```python
from build123d import *

# Parameters (mm, degrees)
CYLINDER_R      = 20
CYLINDER_DEPTH  = 3.3
SKETCH_R        = 1.5
POCKET_DEPTH    = 3.301
POCKET001_DEPTH = 5


with BuildPart() as part:
    # Cylinder → Cylinder (new body)
    with BuildSketch(Plane.XY):
        Circle(CYLINDER_R)
    extrude(amount=CYLINDER_DEPTH)

    # Sketch (on Face2 of Cylinder) → Pocket (cut, through all)
    with BuildSketch(Plane.XY.offset(3.3)):
        with Locations((0, 15.1)):
            Circle(SKETCH_R)
    extrude(amount=-POCKET_DEPTH, mode=Mode.SUBTRACT)

    # CopySketch001 → Pocket001 (cut)
    with BuildSketch(Plane.XY.offset(3.3)):
        Polygon((8.911401, 5.145), (0, 10.29), (-8.911401, 5.145), (-8.911401, -5.145), (0, -10.29), (8.911401, -5.145), align=None)
    extrude(amount=-POCKET001_DEPTH, mode=Mode.SUBTRACT)


solid = part.part
```
The model under review builds one solid part; all positions refer to its coordinate system, in mm. A direction names the side the tool comes from. Coordinates: 2 decimals unless noted, no trailing zeros. Write each loop counter-clockwise with the first axis right and the second up, starting at its lowest first coordinate (ties: lowest second). Pieces come first, ordered by that corner, then holes. Notation, with made-up numbers: (70.5, 83) - (96.5, 83) arc R21 cw to (96.5, 110) - close; hole circle Ø5 at (56, 1.25). An arc over 180 degrees is marked (long way). Answer in a Markdown table with one row per item. Add a question column.
Q1. Consider section B-B on z = 2.4. Give the boundary of the cut face in (x, y) (3 decimals).
Q2. Consider section D-D on x = -17. Give the boundary of the cut face in (y, z).
Q3. To check wall thickness, follow line 1 along Y through (x, z) = (0, 1.6); line 2 along X through (y, z) = (1, 1.55); line 3 along X through (y, z) = (3, 3.15). State the ranges of each line that lie inside material, in increasing order. Write a range as from..to.
Q4. Clearance check with flat-ended pins moving along their axes: pin 1 (1.6 mm diameter, centred on y = -2, z = 2, fed in from -X); pin 2 (1.6 mm diameter, centred on y = -1, z = 2, fed in from +X); pin 3 (1.8 mm diameter, centred on x = 0, y = 15.1, fed in from -Z). State where each tip first meets the part, or that it passes through.
Q5. For faces 1 (the face through (-8.911, 0, 2)), 2 (the face through (-9.2, 0.3, 3.3)), list the 3-axis set-ups (+Z, -Z, +X, -X, +Y, -Y) from which the entire face can be reached by the end or side of a thin tool; tool diameter is ignored.
Q6. Consider section A-A on y = 0. Give the boundary of the cut face in (x, z).
Q7. Draft analysis for pull direction X (two halves, no side actions). For faces 3 (the face through (-9.2, 0.3, 0)), 4 (the face through (-0.195, 16.587, 1.673)), 5 (the face through (-4.336, -19.524, 1.627)), 6 (the face through (-4.393, 7.754, 1.673)), state which applies: +X half, -X half, draft (parallel to the pull), parting line (faces both ways), or undercut.
Q8. Consider section C-C on y = 15.1. Give the boundary of the cut face in (x, z), then the cut area to 3 significant figures.
Answers below:
| question | item | result |
|---|---|---|
| 1 | outline | circle Ø40 at (0, 0); hole (-8.911, -5.145) - (0, -10.29) - (8.911, -5.145) - (8.911, 5.145) - (0, 10.29) - (-8.911, 5.145) - close; hole circle Ø3 at (0, 15.1) |
| 2 | outline | (-10.54, 0) - (10.54, 0) - (10.54, 3.3) - (-10.54, 3.3) - close |
| 3 | line 1 | -20..-10.29, 10.29..13.6, 16.6..20 |
| 3 | line 2 | -19.97..-8.91, 8.91..19.97 |
| 3 | line 3 | -19.77..-8.91, 8.91..19.77 |
| 4 | pin 1 | x = -19.96 |
| 4 | pin 2 | x = 20 |
| 4 | pin 3 | through |
| 5 | face 1 | +Z, -Z |
| 5 | face 2 | +Z, +X, -X, +Y, -Y |
| 6 | outline | (-20, 0) - (-8.91, 0) - (-8.91, 3.3) - (-20, 3.3) - close; (8.91, 0) - (20, 0) - (20, 3.3) - (8.91, 3.3) - close |
| 7 | face 3 | draft |
| 7 | face 4 | undercut |
| 7 | face 5 | parting line |
| 7 | face 6 | undercut |
| 8 | outline | (-13.11, 0) - (-1.5, 0) - (-1.5, 3.3) - (-13.11, 3.3) - close; (1.5, 0) - (13.11, 0) - (13.11, 3.3) - (1.5, 3.3) - close |
| 8 | area | 76.7 mm² |
